CAD build for the part. Positions are in the model's coordinates, mm. Round coordinates to 2 decimals unless told otherwise and drop trailing zeros. Loops run counter-clockwise (first coordinate to the right, second up) from the corner with the lowest first, then second, coordinate; pieces in that order, holes last. Notation, with made-up numbers: M 81.5,-34.5 L 118.5,-34.5 A38 cw 118.5,3.5 Z; hole C 40.5,57 d2. An arc over 180 degrees is marked long. Use one line per item in the form item = value.
from build123d import *

# Parameters (mm, degrees)
F0_R     = 2.6035
F0_R_2   = 12.7
F0_R_3   = 9.525
F1_DEPTH = 590


with BuildPart() as f1:
    # F0 (on Front) → F1 (new body, symmetric)
    with BuildSketch(Plane.XZ):
        Polygon((15.875, -50.8), (25.4, -50.8), (25.4, -41.275), (19.05, -41.275), (19.05, -34.925), (25.4, -34.925), (25.4, -15.875), (19.05, -15.875), (19.05, -9.525), (25.4, -9.525), (25.4, 9.525), (19.05, 9.525), (19.05, 15.875), (25.4, 15.875), (25.4, 34.925), (19.05, 34.925), (19.05, 41.275), (25.4, 41.275), (25.4, 50.8), (15.875, 50.8), (15.875, 44.45), (9.525, 44.45), (9.525, 50.8), (-9.525, 50.8), (-9.525, 44.45), (-15.875, 44.45), (-15.875, 50.8), (-25.4, 50.8), (-25.4, 41.275), (-19.05, 41.275), (-19.05, 34.925), (-25.4, 34.925), (-25.4, 15.875), (-19.05, 15.875), (-19.05, 9.525), (-25.4, 9.525), (-25.4, -9.525), (-19.05, -9.525), (-19.05, -15.875), (-25.4, -15.875), (-25.4, -34.925), (-19.05, -34.925), (-19.05, -41.275), (-25.4, -41.275), (-25.4, -50.8), (-15.875, -50.8), (-15.875, -44.45), (-9.525, -44.45), (-9.525, -50.8), (9.525, -50.8), (9.525, -44.45), (15.875, -44.45), align=None)
        with Locations((-12.7, -38.1)):
            Circle(F0_R, mode=Mode.SUBTRACT)
        with Locations((0, -25.4)):
            Circle(F0_R_2, mode=Mode.SUBTRACT)
        with Locations((-12.7, -12.7)):
            Circle(F0_R, mode=Mode.SUBTRACT)
        Circle(F0_R_3, mode=Mode.SUBTRACT)
        with Locations((12.7, -38.1)):
            Circle(F0_R, mode=Mode.SUBTRACT)
        with Locations((12.7, -12.7)):
            Circle(F0_R, mode=Mode.SUBTRACT)
        with Locations((-12.7, 12.7)):
            Circle(F0_R, mode=Mode.SUBTRACT)
        with Locations((0, 25.4)):
            Circle(F0_R_2, mode=Mode.SUBTRACT)
        with Locations((-12.7, 38.1)):
            Circle(F0_R, mode=Mode.SUBTRACT)
        with Locations((12.7, 12.7)):
            Circle(F0_R, mode=Mode.SUBTRACT)
        with Locations((12.7, 38.1)):
            Circle(F0_R, mode=Mode.SUBTRACT)
    extrude(amount=F1_DEPTH, both=True)


solid = f1.part
1. Drop flat-ended pins along their axis: P1, Ø6, axis at x = -11, y = 114, coming from the +Z side; P2, Ø4.5, axis at x = 12.7, z = 38.1, coming from the +Y side; P3, Ø1.9, axis at x = -13, y = -35, coming from the -Z side; P4, Ø1.9, axis at x = -13.5, y = -226.5, coming from the +Z side. Give the stop position or say it passes through.
Completed:
P1 = 50.8
P2 = through
P3 = -44.45
P4 = 44.45
2. Probe line 1 along Z through (x, y) = (0, 197.5) (3 decimals); line 2 along X through (y, z) = (20, 12); line 3 along Z through (x, y) = (-5.5, -251.5). List the from-to ranges inside material, lowest first. Write a range as from..to.
Completed:
line_1 = -50.8..-38.1, -12.7..-9.525, 9.525..12.7, 38.1..50.8
line_2 = -19.05..-15.21, -10.19..10.19, 15.21..19.05
line_3 = -50.8..-36.85, -13.95..-7.78, 7.78..13.95, 36.85..50.8
3. Cut at A-A on z = -25.4. Write the cut outline in (x, y), and give its area (3 significant figures).
Completed:
outline = M -25.4,-590 L -12.7,-590 L -12.7,590 L -25.4,590 Z; M 12.7,-590 L 25.4,-590 L 25.4,590 L 12.7,590 Z
area = 30,000 mm2
4. Pull direction Z, two halves, no side cores. Call faces 1 (the face through (-7.559, 8.26, -5.796)), 2 (the face through (0, -8, 50.8)), 3 (the face through (25.4, -8, 0)): +Z half, -Z half, draft (parallel to the pull), parting line (faces both ways), or undercut.
Completed:
face_1 = undercut
face_2 = +Z half
face_3 = draft
5. Cut at B-B on y = -513.5. State how many separate pieces and enclosed holes the cut face has, and give its area (3 significant figures).
Completed:
separate_pieces = 1
enclosed_holes = 11
area = 3,210 mm2
